Check sheet for the drawn part. Datum: minimum x, y, z corner. Units: mm. A direction names the side the tool comes from. Round coordinates to 2 decimals unless told otherwise and drop trailing zeros. Write each loop counter-clockwise with the first axis right and the second up, starting at its lowest first coordinate (ties: lowest second). Pieces come first, ordered by that corner, then holes. Notation, with made-up numbers: M -2,73 L 13,73 A12 cw 13,94 Z; hole C 7.5,-9.75 d5. An arc over 180 degrees is marked long. One line per item, written item: value. Start each with the question number.
Item 1: Section check A-A, the plane y = 20.32. Record the cut outline in (x, z), then the cut area to 3 significant figures.
Item 2: Tool access check on the marked faces 4, 5 and 6. Record the directions out of +Z, -Z, +X, -X, +Y, -Y that give a thin tool (end or side, any length) a straight path to the whole face; none if there is none.
Item 3: Section check D-D, the plane y = 14.5. Record the cut outline in (x, z), then the cut area to 3 significant figures.
Item 4: Draft check along Z on the marked faces 1, 2 and 3. Enter one of: +Z half, -Z half, draft (parallel to the pull), parting line (faces both ways), or undercut.
Item 5: Thickness scan on probe 1 along X at (y, z) = (13, 1.75); probe 2 along X at (y, z) = (11.25, 4.25); probe 3 along X at (y, z) = (20.5, 4.25). Record the ranges inside material, lowest first. Write a range as from..to.
Item 6: Section check C-C, the plane x = 25.4. Record the cut outline in (y, z), then the cut area to 3 significant figures.
Item 7: Gauge pin test, flat ends, axial feed: pin 1 (1 mm diameter, centred on x = 11.5, z = 2.5, fed in from -Y); pin 2 (1.8 mm diameter, centred on x = 25.4, y = 20.32, fed in from -Z). Record the tip position at first contact, or that the pin passes through.
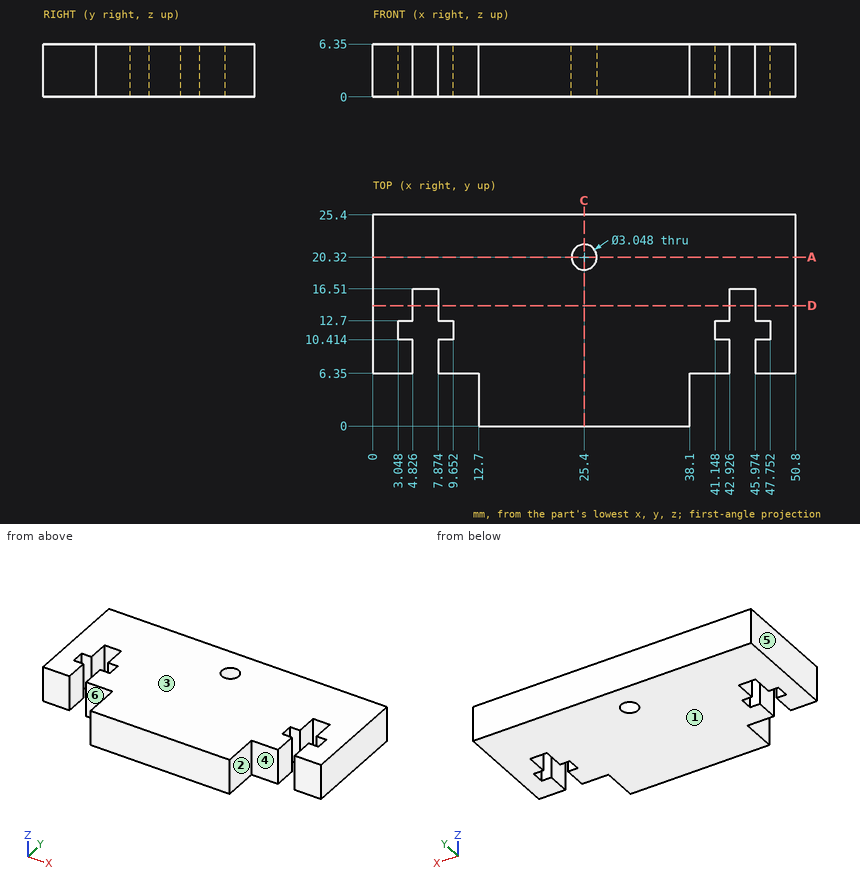
Response values:
1. outline: M 0,0 L 23.88,0 L 23.88,6.35 L 0,6.35 Z; M 26.92,0 L 50.8,0 L 50.8,6.35 L 26.92,6.35 Z
1. area: 303 mm2
2. face 4: +Z, -Z, +X, -Y
2. face 5: +Z, -Z, -X, +Y, -Y
2. face 6: +Z, -Z, -X, -Y
3. outline: M 0,0 L 4.83,0 L 4.83,6.35 L 0,6.35 Z; M 7.87,0 L 42.93,0 L 42.93,6.35 L 7.87,6.35 Z; M 45.97,0 L 50.8,0 L 50.8,6.35 L 45.97,6.35 Z
3. area: 284 mm2
4. face 1: -Z half
4. face 2: draft
4. face 3: +Z half
5. probe 1: x = 0..4.83, 7.87..42.93, 45.97..50.8
5. probe 2: x = 0..3.05, 9.65..41.15, 47.75..50.8
5. probe 3: x = 0..23.89, 26.91..50.8
6. outline: M 0,0 L 18.8,0 L 18.8,6.35 L 0,6.35 Z; M 21.84,0 L 25.4,0 L 25.4,6.35 L 21.84,6.35 Z
6. area: 142 mm2
7. pin 1: stops at y = 6.35
7. pin 2: passes through
